Part model, mm, in its own coordinate system. Face numbers are marked on the shaded views. A direction names the side the tool comes from. Coordinates: 2 decimals unless noted, no trailing zeros. Order: outer loops, then holes, each group sorted by start corner. A loop starts at its lowest first (then second) coordinate and runs counter-clockwise, first axis right, second up.
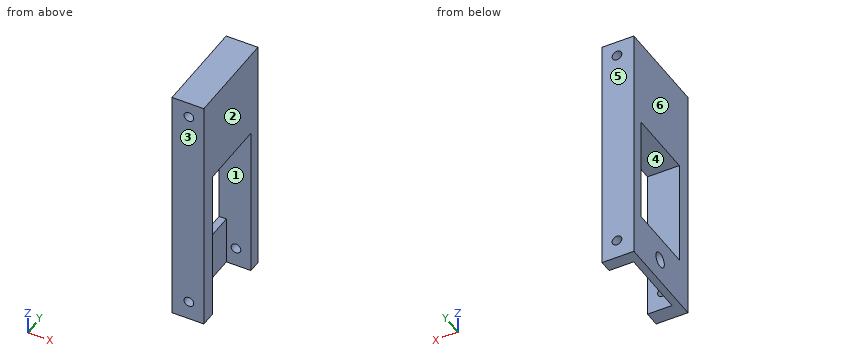
Autodesk Inventor part; units mm, degrees
ref_plane "YZ Plane" through (0, 0, 0) normal (1, 0, 0) x (0, 1, 0)
ref_plane "XZ Plane" through (0, 0, 0) normal (0, 1, 0) x (-1, 0, 0)
ref_plane "XY Plane" through (0, 0, 0) normal (0, 0, 1) x (1, 0, 0)
sketch "Эскиз1" plane through (0, 0, 0) normal (0, 1, 0) x (-1, 0, 0)
  circle A0 centre (0, 21.0368) radius 1
  circle A1 centre (0, -22.0362) radius 1
  line L0 (3.4815, 24.1933) -> (-3.0824, 24.1933)
  line L1 (-3.0824, 24.1933) -> (-3.0824, -25.9673)
  line L2 (-3.0824, -25.9673) -> (3.4815, -25.9673)
  line L3 (3.4815, -25.9673) -> (3.4815, 24.1933)
  point P0 (0, 0)
  dimension "d0" = 43.073
  dimension "d1" = 2
  dimension "d2" = 2
extrude "Выдавливание1" add sketch "Эскиз1" along normal blind 20
sketch "Эскиз2" plane through (3.0824, 0, 24.1933) normal (1, 0, 0) x (0, 0, -1)
  line L0 (50.1606, 0) -> (50.1606, 20)
  line L1 (0, 0) -> (0, 20)
  line L2 (50.1606, 17.3924) -> (0, 17.3924)
  line L3 (0, 17.3924) -> (0, 3.1924)
  line L4 (0, 3.1924) -> (50.1606, 3.1924)
  line L5 (50.1606, 3.1924) -> (50.1606, 17.3924)
  line L6 (18.1606, 3.1924) -> (18.1606, 17.3924)
  line L7 (40.1606, 17.3924) -> (40.1606, 3.1924)
  line L8 (45.2295, 20) -> (45.2295, 0)
  circle A0 centre (45.2295, 10.2924) radius 1.55
  point P0 (24.1933, 0)
  point P1 (50.1606, 10)
  dimension "d5" = 14.2
  dimension "d6" = 32
  dimension "d7" = 10
  dimension "d8" = 3.1
extrude "Выдавливание2" cut sketch "Эскиз2" against normal through all contours L4 L6 L2 L7 | A0 L8 | L8 A0
extrude "Выдавливание3" cut sketch "Эскиз2" against normal blind 5.064 contours L4 L8 A0 L2 L0 | L4 L7 L2 L8 A0
properties part number "tcrt_to_mgn7"
(1) Slice it at D-D, the plane z = -18.5. Give the cut face in (x, y), then the cut area to 3 significant figures.
(2) Tool access for the marked faces 1 and 2: list every direction of +Z, -Z, +X, -X, +Y, -Y with a clear straight run to the whole face (end or side of a thin tool).
(3) Probe line 1 (Z direction, x = 0, y = 19.05); line 2 (Y direction, x = 0, z = 2); line 3 (Z direction, x = -3, y = 16.25). List the from-to ranges inside material, lowest first.
(4) Slice it at C-C, the plane y = 7.75. Give the cut face in (x, z).
(5) Slice it at A-A, the plane z = 5. Give the cut face in (x, y), then the cut area to 3 significant figures.
(6) Drop flat-ended pins along their axis: pin 1 (1.2 mm diameter, centred on x = 0, z = 21.04, fed in from -Y); pin 2 (2 mm diameter, centred on x = 1, y = 10.5, fed in from -Z); pin 3 (5 mm diameter, centred on y = 12, z = -21, fed in from +X). Give the stop position or say it passes through.
(7) Pull direction Y, two halves, no side cores. Call the marked faces 3, 4, 5 and 6: +Y half, -Y half, draft (parallel to the pull), parting line (faces both ways), or undercut.
(8) Slice it at B-B, the plane x = 0. Give the cut face in (y, z), then the cut area to 3 significant figures.
Here are the results:
1. outline: (-3.48, 0) - (3.08, 0) - (3.08, 3.19) - (-1.98, 3.19) - (-1.98, 17.39) - (3.08, 17.39) - (3.08, 20) - (-3.48, 20) - close
1. area: 59.4 mm2
2. face 1: +X
2. face 2: +Z, -Z, +X, +Y, -Y
3. line 1: z = -25.97 to -23.04, -21.04 to 20.04, 22.04 to 24.19
3. line 2: y = 0 to 3.19, 17.39 to 20
3. line 3: z = -25.97 to -15.97, 6.03 to 24.19
4. outline: (-3.48, -25.97) - (-1.98, -25.97) - (-1.98, -15.97) - (-3.48, -15.97) - close; (-3.48, 6.03) - (3.08, 6.03) - (3.08, 24.19) - (-3.48, 24.19) - close; hole circle Ø2 at (0, 21.04)
5. outline: (-3.48, 0) - (3.08, 0) - (3.08, 3.19) - (-3.48, 3.19) - close; (-3.48, 17.39) - (3.08, 17.39) - (3.08, 20) - (-3.48, 20) - close
5. area: 38.1 mm2
6. pin 1: passes through
6. pin 2: stops at z = 6.03
6. pin 3: stops at x = -1.98
7. face 3: -Y half
7. face 4: undercut
7. face 5: +Y half
7. face 6: draft
8. outline: (0, -25.97) - (3.19, -25.97) - (3.19, -23.04) - (0, -23.04) - close; (0, -21.04) - (3.19, -21.04) - (3.19, 6.03) - (17.39, 6.03) - (17.39, -21.04) - (20, -21.04) - (20, 20.04) - (0, 20.04) - close; (0, 22.04) - (20, 22.04) - (20, 24.19) - (0, 24.19) - close; (17.39, -25.97) - (20, -25.97) - (20, -23.04) - (17.39, -23.04) - close
8. area: 497 mm2
